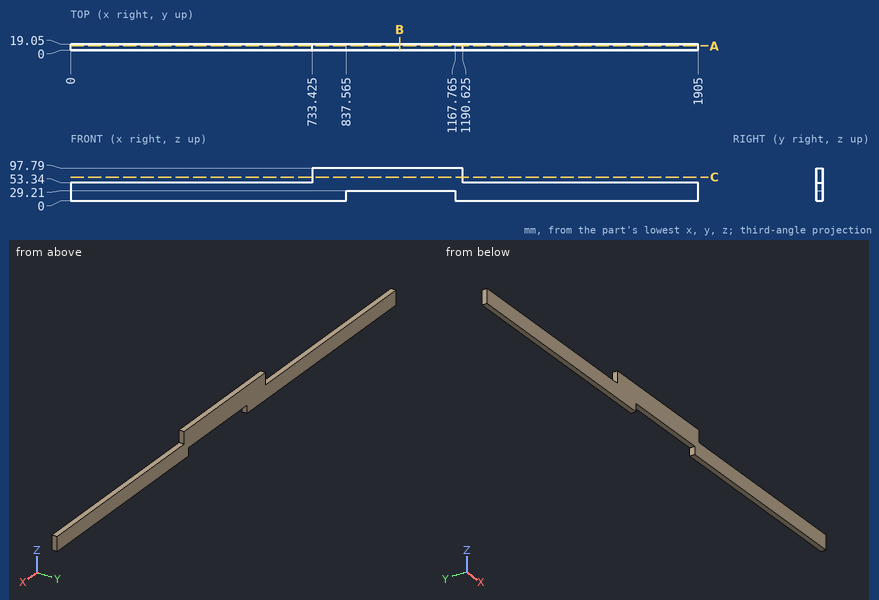
The drawing under review shows one solid part. Ordinate dimensions are in mm from its lowest x, y, z. Give positions to 0.01 mm unless a question says otherwise; leave off trailing zeros. Order: outer loops, then holes, each group sorted by start corner. A loop starts at its lowest first (then second) coordinate and runs counter-clockwise, first axis right, second up. Notation, with made-up numbers: (16.25, 31) -> (21.25, 31) arc R16 cw to (21.25, 50) -> close; hole circle Ø10 at (35.5, 15.25). An arc over 180 degrees is marked (long way). Write item = value, one per line. Start each with the question number.
(1) We need section A-A on y = 13. Write out the cut boundary in (x, z) (3 decimals).
(2) We need section B-B on x = 998.5. Write out the cut boundary in (y, z), plus the area to 3 significant figures.
(3) To check wall thickness, follow line 1 along X through (y, z) = (3.75, 26.5) (3 decimals); line 2 along Z through (x, y) = (1152, 15.5); line 3 along X through (y, z) = (9.25, 65) (3 decimals). State the ranges of each line that lie inside material, in increasing order.
(4) We need section C-C on z = 71. Write out the cut boundary in (x, y) (3 decimals), plus the area to 3 significant figures.
(5) For pin 1 (3 mm diameter, centred on x = 290, y = 12.5, fed in from +Z); pin 2 (8 mm diameter, centred on y = 2.5, z = 58.5, fed in from -X) (3 decimals), all flat-tipped, find the tip position at first contact; note any pin that passes through.
Numbers:
q1.outline = (0, 0) -> (837.565, 0) -> (837.565, 29.21) -> (1167.765, 29.21) -> (1167.765, 0) -> (1905, 0) -> (1905, 53.34) -> (1190.625, 53.34) -> (1190.625, 97.79) -> (733.425, 97.79) -> (733.425, 53.34) -> (0, 53.34) -> close
q2.outline = (0, 29.21) -> (19.05, 29.21) -> (19.05, 97.79) -> (0, 97.79) -> close
q2.area = 1,310 mm^2
q3.line_1 = 0 to 837.565, 1167.765 to 1905
q3.line_2 = 29.21 to 97.79
q3.line_3 = 733.425 to 1190.625
q4.outline = (733.425, 0) -> (1190.625, 0) -> (1190.625, 19.05) -> (733.425, 19.05) -> close
q4.area = 8,710 mm^2
q5.pin_1 = 53.34
q5.pin_2 = 733.425
